Study the drawing (mm; zero at the part's minimum x, y, z) and answer. A direction names the side the tool comes from. Coordinates: 2 decimals unless noted, no trailing zeros. Loops run counter-clockwise (first coordinate to the right, second up) from the corner with the lowest first, then second, coordinate; pieces in that order, holes last.
Q1. Straight lines are drawn through the part: line 1 (Y direction, x = 56, z = 16); line 2 (Y direction, x = 5.5, z = 71.5); line 3 (Z direction, x = 4.5, y = 54). For each, find the intervals that lie inside material, in ascending order.
Q2. Section B-B (z = 37.5) is taken. Give the vertices of the cut face in (x, y), then the cut area to 3 significant figures.
Q3. Section C-C (x = 26) is taken. Give the vertices of the cut face in (y, z).
Q4. Which of the six approach directions +Z, -Z, +X, -X, +Y, -Y give full straight-line access (tool end or side, diameter ignored) to the marked faces 1 and 2?
Q5. Section A-A (x = 37.5) is taken. Give the vertices of the cut face in (y, z).
Q6. Flat-ended cylindrical pins translate along their axes: P1, Ø3, axis at x = 12.5, z = 59, coming from the -Y side; P2, Ø8, axis at y = 19.5, z = 42, coming from the -X side. Find the tip coordinate at first contact, or state that the pin passes through.
Q7. Section D-D (z = 30) is taken. Give the vertices of the cut face in (x, y).
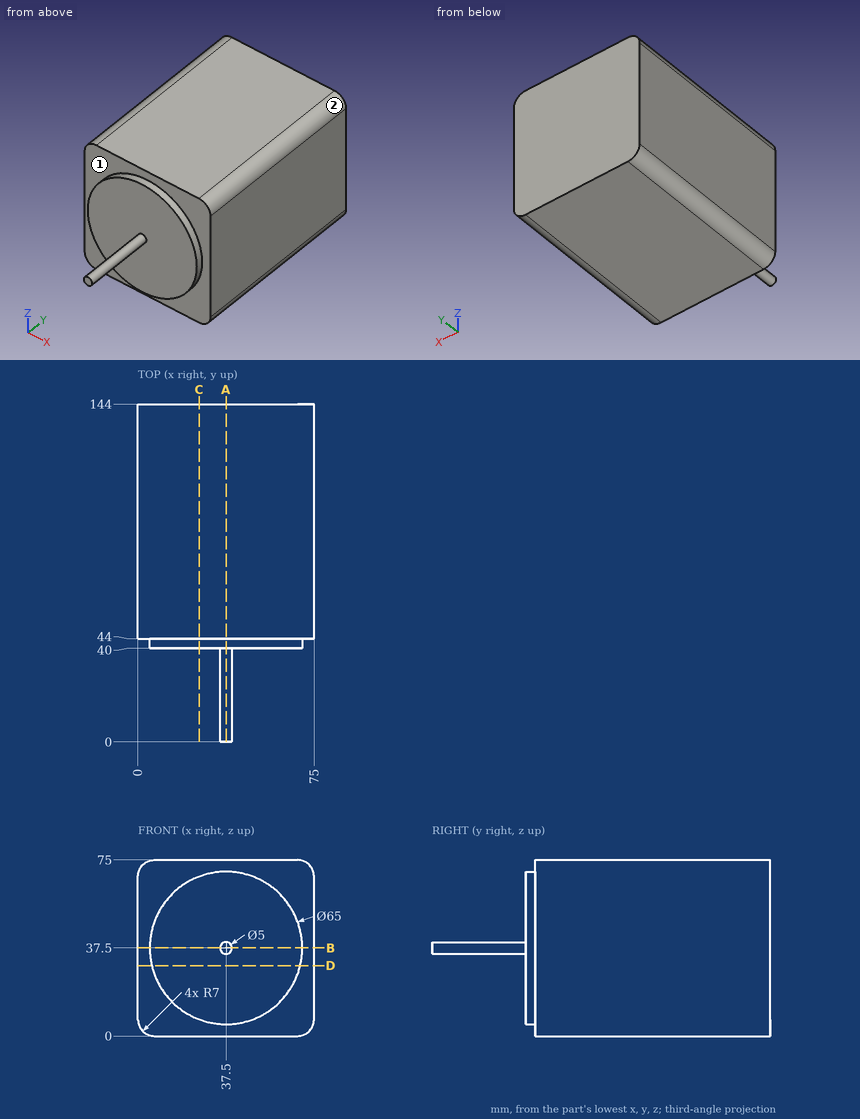
Numbers:
1. line 1: y = 40 to 144
1. line 2: y = 44 to 144
1. line 3: z = 0.46 to 74.54
2. outline: (0, 44) - (5, 44) - (5, 40) - (35, 40) - (35, 0) - (40, 0) - (40, 40) - (70, 40) - (70, 44) - (75, 44) - (75, 144) - (0, 144) - close
2. area: 7,960 mm2
3. outline: (40, 7.1) - (44, 7.1) - (44, 0) - (144, 0) - (144, 75) - (44, 75) - (44, 67.9) - (40, 67.9) - close
4. face 1: -Y
4. face 2: +Z, +X, +Y, -Y
5. outline: (0, 35) - (40, 35) - (40, 5) - (44, 5) - (44, 0) - (144, 0) - (144, 75) - (44, 75) - (44, 70) - (40, 70) - (40, 40) - (0, 40) - close
6. P1: stops at y = 40
6. P2: stops at x = 35.05
7. outline: (0, 44) - (5.88, 44) - (5.88, 40) - (69.12, 40) - (69.12, 44) - (75, 44) - (75, 144) - (0, 144) - close
